Could you check a few things on this drawing? It's one solid part, dimensions in mm from its lowest x, y, z. Round coordinates to 2 decimals unless told otherwise and drop trailing zeros. Write each loop counter-clockwise with the first axis right and the second up, starting at its lowest first coordinate (ties: lowest second). Pieces come first, ordered by that corner, then holes. Notation, with made-up numbers: (83, 24.25) -> (107, 24.25) arc R34 cw to (107, 58.25) -> close; hole circle Ø2 at (-27, 61). An arc over 180 degrees is marked (long way). Return JSON: item names as keys, results as strings.
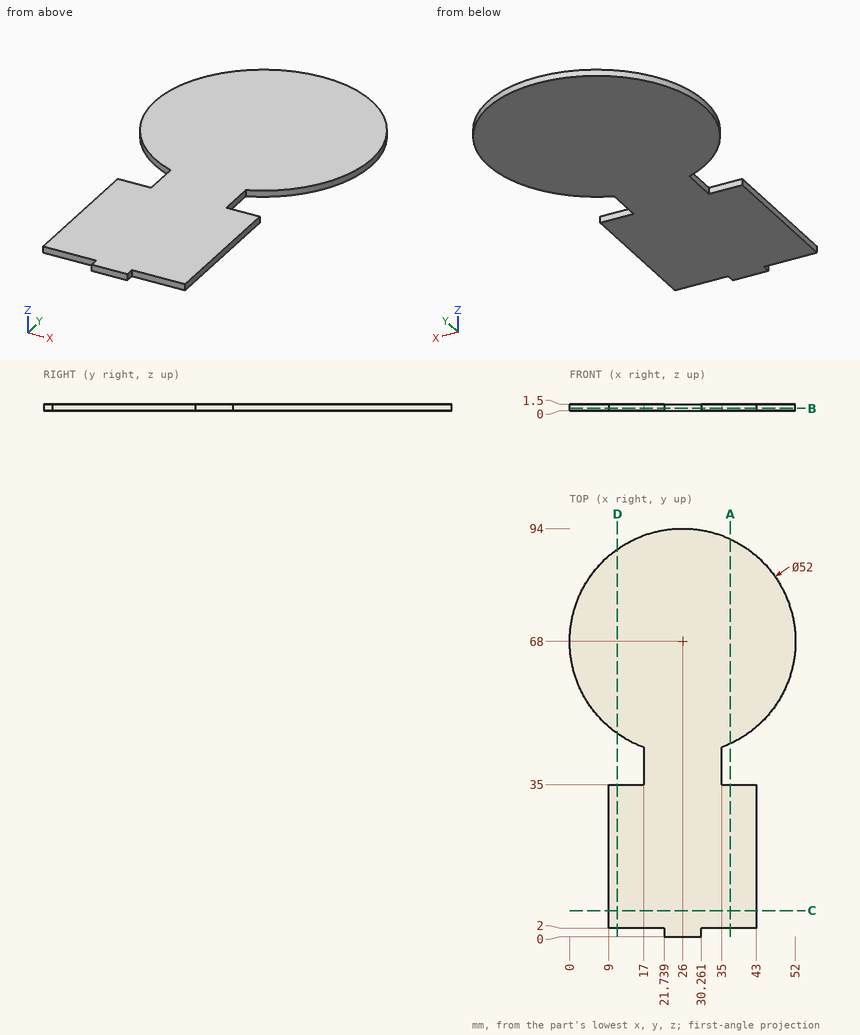
1) I want a section at D-D, the plane x = 11. Please give me the cut outline in (y, z).
Return value:
{"outline": "(2, 0) -> (35, 0) -> (35, 1.5) -> (2, 1.5) -> close; (46.76, 0) -> (89.24, 0) -> (89.24, 1.5) -> (46.76, 1.5) -> close"}
2) I want a section at C-C, the plane y = 6. Please give me the cut outline in (x, z), and give its area (3 significant figures).
Return value:
{"outline": "(9, 0) -> (43, 0) -> (43, 1.5) -> (9, 1.5) -> close", "area": "51.0 mm²"}
3) I want a section at A-A, the plane x = 37. Please give me the cut outline in (y, z).
Return value:
{"outline": "(2, 0) -> (35, 0) -> (35, 1.5) -> (2, 1.5) -> close; (44.44, 0) -> (91.56, 0) -> (91.56, 1.5) -> (44.44, 1.5) -> close"}
4) If I drill on probe 1 along X at (y, z) = (39, 1.25); probe 2 along Y at (x, z) = (14.5, 1.1); probe 3 along X at (y, z) = (7, 0.6), over which ranges is the centre line in solid material (lowest first)? Write a range as [from, to].
Return value:
{"probe 1": "[17, 35]", "probe 2": "[2, 35], [44.68, 91.32]", "probe 3": "[9, 43]"}
5) Will these pins go through, and if not, where does the flat tip stop? pin 1 Ø0.8 at (x, z) = (41, 0.5) entering from +Y; pin 2 Ø0.8 at (x, z) = (15, 1) entering from -Y; pin 3 Ø1 at (x, y) = (31.5, 35) entering from -Z; pin 4 Ø0.8 at (y, z) = (13.5, 0.5) entering from +X.
Return value:
{"pin 1": "y = 89.51", "pin 2": "y = 2", "pin 3": "z = 0", "pin 4": "x = 43"}
6) I want a section at B-B, the plane z = 0.5. Please give me the cut outline in (x, y), and give its area (3 significant figures).
Return value:
{"outline": "(9, 2) -> (21.74, 2) -> (21.74, 0) -> (30.26, 0) -> (30.26, 2) -> (43, 2) -> (43, 35) -> (35, 35) -> (35, 43.61) arc R26 ccw (long way) to (17, 43.61) -> (17, 35) -> (9, 35) -> close", "area": "3,400 mm²"}
